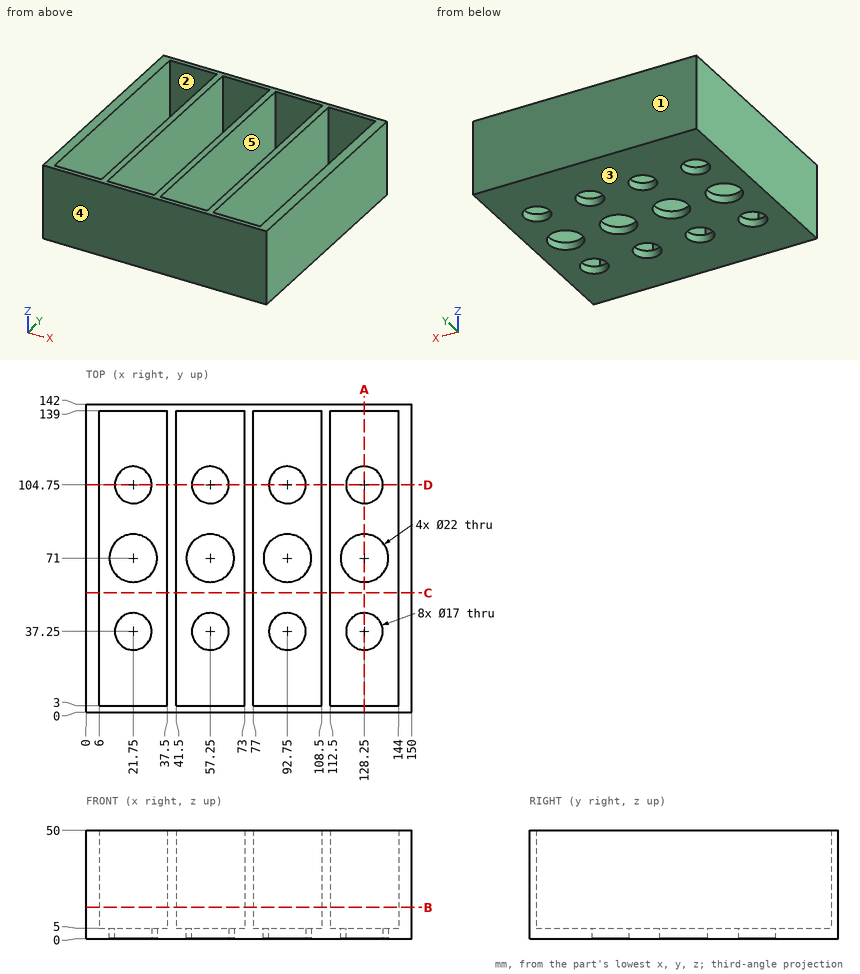
The figure shows three views and two pictorial views of one solid part (mm, origin at its lowest corner). Answer the questions. A direction names the side the tool comes from. Round coordinates to 2 decimals unless told otherwise and drop trailing zeros. Loops run counter-clockwise (first coordinate to the right, second up) from the corner with the lowest first, then second, coordinate; pieces in that order, holes last. Notation, with made-up numbers: M 88.25,60 L 134.25,60 A17 cw 134.25,86 Z; hole C -3,38 d10. An arc over 180 degrees is marked long. Write each question's results on one line, items separated by ' | '. Start each with the question number.
1) Find section B-B on z = 14.5. Write down the section's boundary in (x, y), plus the area to 3 significant figures.
2) Straight lines are drawn through the part: probe 1 along X at (y, z) = (55.5, 36); probe 2 along Y at (x, z) = (128, 3); probe 3 along X at (y, z) = (104, 3). For each, find the intervals that lie inside material, in ascending order.
3) Find section A-A on x = 128.25. Write down the section's boundary in (y, z), plus the area to 3 significant figures.
4) Determine the mould class of the marked faces 1, 2 and 3 for opening direction Y: pulls with the +Y half, pulls with the -Y half, needs draft (parallel to the pull), parting line crosses it, or undercut.
5) Find section D-D on y = 104.75. Count the separate pieces of the cut face and the enclosed holes in it, plus the area to 3 significant figures.
6) Find section C-C on y = 55. Write down the section's boundary in (x, z).
7) Each of these flat-tipped pins is pushed along its axis until it touches: pin 1 (16 mm diameter, centred on x = 62.5, y = 40.5, fed in from +Z); pin 2 (13.5 mm diameter, centred on x = 128.25, y = 37.25, fed in from +Z). Where does it stop, or does it pass through?
8) Which of the six approach directions +Z, -Z, +X, -X, +Y, -Y give full straight-line access (tool end or side, diameter ignored) to the marked faces 4 and 5?
Final values:
1) outline: M 0,0 L 150,0 L 150,142 L 0,142 Z; hole M 6,3 L 37.5,3 L 37.5,139 L 6,139 Z; hole M 41.5,3 L 73,3 L 73,139 L 41.5,139 Z; hole M 77,3 L 108.5,3 L 108.5,139 L 77,139 Z; hole M 112.5,3 L 144,3 L 144,139 L 112.5,139 Z | area: 4,160 mm²
2) probe 1: 0 to 6, 37.5 to 41.5, 73 to 77, 108.5 to 112.5, 144 to 150 | probe 2: 0 to 28.75, 45.75 to 60, 82 to 96.25, 113.25 to 142 | probe 3: 0 to 13.28, 30.22 to 48.78, 65.72 to 84.28, 101.22 to 119.78, 136.72 to 150
3) outline: M 0,0 L 28.75,0 L 28.75,5 L 3,5 L 3,50 L 0,50 Z; M 45.75,0 L 60,0 L 60,5 L 45.75,5 Z; M 82,0 L 96.25,0 L 96.25,5 L 82,5 Z; M 113.25,0 L 142,0 L 142,50 L 139,50 L 139,5 L 113.25,5 Z | area: 700 mm²
4) face 1: pulls with the +Y half | face 2: undercut | face 3: needs draft
5) separate pieces: 5 | enclosed holes: 0 | area: 1,490 mm²
6) outline: M 0,0 L 150,0 L 150,50 L 144,50 L 144,5 L 112.5,5 L 112.5,50 L 108.5,50 L 108.5,5 L 77,5 L 77,50 L 73,50 L 73,5 L 41.5,5 L 41.5,50 L 37.5,50 L 37.5,5 L 6,5 L 6,50 L 0,50 Z
7) pin 1: z = 5 | pin 2: through
8) face 4: +Z, -Z, +X, -X, -Y | face 5: +Z
